Autodesk Inventor part; units mm, degrees
ref_plane "YZ Plane" through (0, 0, 0) normal (1, 0, 0) x (0, 1, 0)
ref_plane "XZ Plane" through (0, 0, 0) normal (0, 1, 0) x (-1, 0, 0)
ref_plane "XY Plane" through (0, 0, 0) normal (0, 0, 1) x (1, 0, 0)
sketch "Sketch1" plane through (0, 0, 0) normal (0, 1, 0) x (-1, 0, 0)
  circle A0 centre (0, 0) radius 12.7
  dimension "d0" = 25.4
extrude "Extrusion1" add sketch "Sketch1" along normal blind 180
sketch "Sketch3" plane through (0, 180, 0) normal (0, 1, 0) x (1, 0, 0)
  point P0 (0, 0)
  point P1 (0, 0)
hole "Hole2" at (0, 180, 0) direction (0, -1, 0) diameter 10 end through all
sketch "Sketch4" plane through (0, 180, 0) normal (0, 1, 0) x (1, 0, 0)
  point P0 (0, 0)
  point P1 (0, -8.25)
  point P2 (-8.25, 0)
  point P3 (0, 8.25)
  point P4 (8.25, 0)
  dimension "d17" = 8.25
  dimension "d20" = 360
hole "Hole3" at (0, 180, 8.25) at (-8.25, 180, 0) at (0, 180, -8.25) at (8.25, 180, 0) direction (0, -1, 0) diameter 3 depth 38.1 tip angle 118
thread "Thread1"
thread "Thread2"
thread "Thread3"
thread "Thread4"
sketch "Sketch5" plane through (0, 0, 0) normal (0, -1, 0) x (1, 0, 0)
  circle A0 centre (8.25, 0) radius 1.5
  circle A1 centre (0, 8.25) radius 1.5
  circle A2 centre (-8.25, 0) radius 1.5
  circle A3 centre (0, -8.25) radius 1.5
  point P0 (0, 0)
hole "Hole4" at (8.25, 0, 0) at (0, 0, 8.25) at (-8.25, 0, 0) at (0, 0, -8.25) direction (0, 1, 0) diameter 3 depth 25.4
thread "Thread5"
thread "Thread6"
thread "Thread7"
thread "Thread8"
properties part number "BarraSolidaMotor"
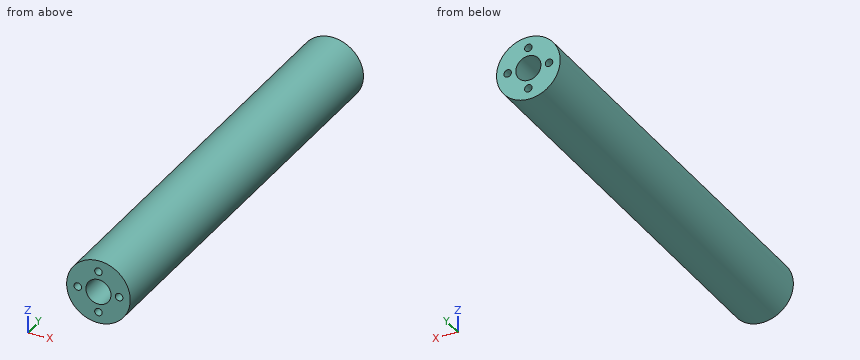
Model file for the job. Use its own axes, mm. Round coordinates to 2 decimals unless told otherwise and drop trailing zeros. Order: outer loops, then holes, each group sorted by start corner. A loop starts at its lowest first (then second) coordinate and runs counter-clockwise, first axis right, second up. Notation, with made-up numbers: M 8,70 L 12,70 A21 cw 12,97 Z; hole C 40.25,37.5 d4. An arc over 180 degrees is marked long. Write each question's results on one line, items separated by ' | '. Start each with the question number.
(1) Probe probe 1 along Z at (x, y) = (0, 171); probe 2 along X at (y, z) = (165, -0.75); probe 3 along X at (y, z) = (71, 2.75). List the from-to ranges inside material, lowest first. Write a range as from..to.
(2) Saw through at A-A, the plane y = 145. Give the cut face in (x, z).
(3) Drop flat-ended pins along their axis: pin 1 (12 mm diameter, centred on x = -8.5, y = 63.5, fed in from -Z); pin 2 (0.9 mm diameter, centred on x = -8, z = -0.5, fed in from -Y); pin 3 (1 mm diameter, centred on x = -7.5, y = 28.5, fed in from -Z). Give the stop position or say it passes through.
(4) Saw through at B-B, the plane y = 57. Give the cut face in (x, z).
Established:
1) probe 1: z = -12.7..-9.75, -6.75..-5, 5..6.75, 9.75..12.7 | probe 2: x = -12.68..-9.55, -6.95..-4.94, 4.94..6.95, 9.55..12.68 | probe 3: x = -12.4..-4.18, 4.18..12.4
2) outline: C 0,0 d25.4; hole C -8.25,0 d3; hole C 0,0 d10; hole C 0,-8.25 d3; hole C 0,8.25 d3; hole C 8.25,0 d3
3) pin 1: stops at z = -12.45 | pin 2: stops at y = 25.4 | pin 3: stops at z = -10.6
4) outline: C 0,0 d25.4; hole C 0,0 d10
